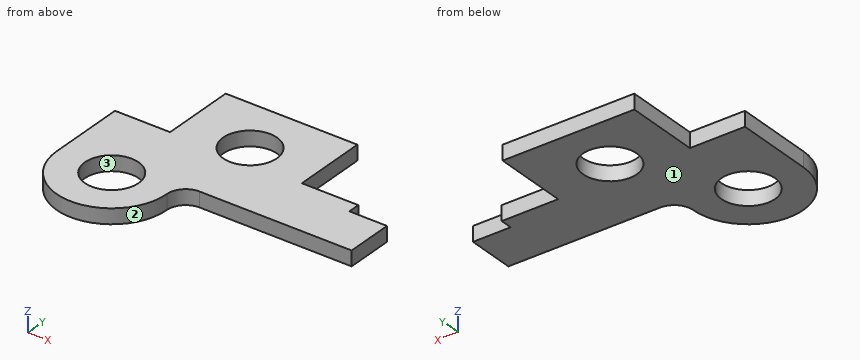
from build123d import *

# Parameters (mm, degrees)
SKETCH1_R           = 14.2875
BOSS_EXTRUDE1_DEPTH = 7.9375


with BuildPart() as part:
    # Sketch1 → Boss-Extrude1 (new body)
    with BuildSketch(Plane.XY):
        with BuildLine():
            Line((149.2875, 39.2875), (149.2875, 64.4375))
            Line((149.2875, 64.4375), (129.2875, 64.4375))
            Line((129.2875, 64.4375), (129.2875, 70.7875))
            Line((129.2875, 70.7875), (99.2875, 70.7875))
            Line((99.2875, 70.7875), (99.2875, 110.2875))
            Line((99.2875, 110.2875), (29.2875, 110.2875))
            Line((29.2875, 110.2875), (29.2875, 70.7875))
            Line((29.2875, 70.7875), (0, 70.7875))
            Line((0, 70.7875), (0, 29.2875))
            ThreePointArc((0, 29.2875), (29.2875, 0), (58.575, 29.2875))
            ThreePointArc((58.575, 29.2875), (61.503932188, 36.358567812), (68.575, 39.2875))
            Line((68.575, 39.2875), (149.2875, 39.2875))
        make_face()
        with Locations((64.2875, 80.7875)):
            Circle(SKETCH1_R, mode=Mode.SUBTRACT)
        with Locations((29.2875, 29.2875)):
            Circle(SKETCH1_R, mode=Mode.SUBTRACT)
    extrude(amount=BOSS_EXTRUDE1_DEPTH)


solid = part.part
Read the model definition and answer for the solid it produces. Units are mm, in the model's axes. Face numbers are marked on the shaded views. Give positions to 0.01 mm unless a question says otherwise; leave off trailing zeros. Loops run counter-clockwise (first coordinate to the right, second up) from the corner with the lowest first, then second, coordinate; pieces in that order, holes last. Notation, with made-up numbers: (-25.75, 57) -> (20.25, 57) arc R24 ccw to (20.25, 72) -> close; hole circle Ø10 at (-28, -5). An arc over 180 degrees is marked (long way). Use a Markdown table: item, result.
Q1. Each of these flat-tipped pins is pushed along its axis until it touches: pin 1 (4 mm diameter, centred on x = 139.5, z = 5, fed in from +Y); pin 2 (2.5 mm diameter, centred on x = 124, z = 5, fed in from -Y); pin 3 (1 mm diameter, centred on y = 72, z = 4, fed in from +X). Where does it stop, or does it pass through?
Solved:
| item | result |
|---|---|
| pin 1 | stops at y = 64.44 |
| pin 2 | stops at y = 39.29 |
| pin 3 | stops at x = 99.29 |
Q2. Determine the mould class of the marked faces 1, 2 and 3 for opening direction X: pulls with the +X half, pulls with the -X half, needs draft (parallel to the pull), parting line crosses it, or undercut.
Solved:
| item | result |
|---|---|
| face 1 | needs draft |
| face 2 | parting line crosses it |
| face 3 | undercut |
Q3. Section C-C, the plane z = 4.75 is taken. Determine the outline of the cut face in (x, y) (1 decimal), then the cut area to 3 significant figures.
Solved:
| item | result |
|---|---|
| outline | (0, 29.3) arc R29.3 ccw to (58.6, 29.3) arc R10 cw to (68.6, 39.3) -> (149.3, 39.3) -> (149.3, 64.4) -> (129.3, 64.4) -> (129.3, 70.8) -> (99.3, 70.8) -> (99.3, 110.3) -> (29.3, 110.3) -> (29.3, 70.8) -> (0, 70.8) -> close; hole circle Ø28.6 at (29.3, 29.3); hole circle Ø28.6 at (64.3, 80.8) |
| area | 8,010 mm^2 |
Q4. Section A-A, the plane y = 34 is taken. Determine the outline of the cut face in (x, z) (1 decimal), then the cut area to 3 significant figures.
Solved:
| item | result |
|---|---|
| outline | (0, 0) -> (15.8, 0) -> (15.8, 7.9) -> (0, 7.9) -> close; (42.8, 0) -> (59.8, 0) -> (59.8, 7.9) -> (42.8, 7.9) -> close |
| area | 260 mm^2 |
Q5. Find the intervals of material crossed by line 1 along Y through (x, z) = (28.5, 1.5); line 2 along Y through (x, z) = (104, 2.5); line 3 along X through (y, z) = (87, 7.5), in increasing order.
Solved:
| item | result |
|---|---|
| line 1 | y = 0.01 to 15.02, 43.55 to 70.79 |
| line 2 | y = 39.29 to 70.79 |
| line 3 | x = 29.29 to 51.42, 77.15 to 99.29 |
Q6. Section D-D, the plane x = 121 is taken. Determine the outline of the cut face in (y, z), then the cut area to 3 significant figures.
Solved:
| item | result |
|---|---|
| outline | (39.29, 0) -> (70.79, 0) -> (70.79, 7.94) -> (39.29, 7.94) -> close |
| area | 250 mm^2 |
Q7. Section B-B, the plane x = 56.5 is taken. Determine the outline of the cut face in (y, z), then the cut area to 3 significant figures.
Solved:
| item | result |
|---|---|
| outline | (18.46, 0) -> (68.81, 0) -> (68.81, 7.94) -> (18.46, 7.94) -> close; (92.77, 0) -> (110.29, 0) -> (110.29, 7.94) -> (92.77, 7.94) -> close |
| area | 539 mm^2 |
